from build123d import *

# Parameters (mm, degrees)
SKETCH_1_R      = 0.75
EXTRUDE_1_DEPTH = 15
SKETCH_3_R      = 0.75
EXTRUDE_2_DEPTH = 2
SKETCH_5_R      = 0.75
EXTRUDE_3_DEPTH = 25
SKETCH_7_R      = 0.75
EXTRUDE_4_DEPTH = 5
EXTRUDE_START   = 25
SKETCH_9_R      = 0.75
EXTRUDE_5_DEPTH = 6


with BuildPart() as part:
    # 草图1 → 凸台-拉伸1 (new body)
    with BuildSketch(Plane(origin=(0, 0, 0), x_dir=(1, 0, 0), z_dir=(0, 1, 0))):
        with Locations(Location((0, 0, 0), (0, 0, 270))):
            Circle(SKETCH_1_R)
    extrude(amount=EXTRUDE_1_DEPTH)

    # 草图2 → 旋转1 (revolve)
    with BuildSketch(Plane.XY):
        with BuildLine():
            Line((0, 15.75), (0, 14.25))
            ThreePointArc((0, 14.25), (0.75, 15), (0, 15.75))
        make_face()
    revolve(axis=Axis((0, 15.75, 0), (0, -1, 0)))

    # 草图3 → 凸台-拉伸2 (add)
    with BuildSketch(Plane(origin=(0, 0, 0), x_dir=(0, 0, -1), z_dir=(1, 0, 0))):
        with Locations((0, 15)):
            Circle(SKETCH_3_R)
    extrude(amount=EXTRUDE_2_DEPTH)

    # 草图4 → 旋转2 (revolve)
    with BuildSketch(Plane(origin=(2, 0, 0), x_dir=(0, 0, -1), z_dir=(1, 0, 0))):
        with BuildLine():
            Line((0, 15.75), (0, 14.25))
            ThreePointArc((0, 14.25), (0.75, 15), (0, 15.75))
        make_face()
    revolve(axis=Axis((2, 15.75, 0), (0, -1, 0)))

    # 草图5 → 凸台-拉伸3 (add)
    with BuildSketch(Plane(origin=(0, 15, 0), x_dir=(1, 0, 0), z_dir=(0, 1, 0))):
        with Locations(Location((2, 0, 0), (0, 0, 270))):
            Circle(SKETCH_5_R)
    extrude(amount=EXTRUDE_3_DEPTH)

    # 草图6 → 旋转3 (revolve)
    with BuildSketch(Plane(origin=(0, 40, 0), x_dir=(1, 0, 0), z_dir=(0, 1, 0))):
        with BuildLine():
            Line((2, 0.75), (2, -0.75))
            ThreePointArc((2, -0.75), (2.75, 0), (2, 0.75))
        make_face()
    revolve(axis=Axis((2, 40, -0.75), (0, 0, 1)))

    # 草图7 → 凸台-拉伸4 (add)
    with BuildSketch(Plane(origin=(2, 0, 0), x_dir=(0, 0, -1), z_dir=(1, 0, 0))):
        with Locations((0, 40)):
            Circle(SKETCH_7_R)
    extrude(amount=-EXTRUDE_4_DEPTH)

    # 草图8 → 旋转5 (revolve)
    with BuildSketch(Plane.ZY.offset(3)):
        with BuildLine():
            Line((-0.75, 40), (0.75, 40))
            ThreePointArc((0.75, 40), (0, 40.75), (-0.75, 40))
        make_face()
    revolve(axis=Axis((-3, 40, -0.75), (0, 0, 1)))

    # 草图9 → 凸台-拉伸5 (add)
    with BuildSketch(Plane(origin=(0, 15, 0), x_dir=(1, 0, 0), z_dir=(0, 1, 0)).offset(EXTRUDE_START)):
        with Locations(Location((-3, 0, 0), (0, 0, 270))):
            Circle(SKETCH_9_R)
    extrude(amount=EXTRUDE_5_DEPTH)


solid = part.part
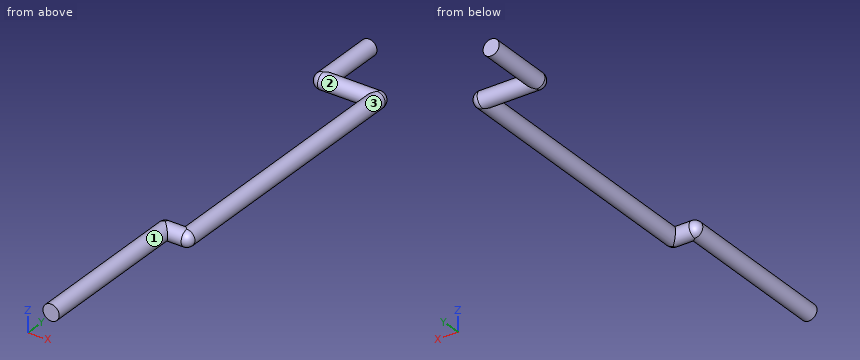
Could you check a few things on this model? Use its own coordinates, in mm. Face numbers are marked on the shaded views. Round coordinates to 2 decimals unless told otherwise and drop trailing zeros. Loops run counter-clockwise (first coordinate to the right, second up) from the corner with the lowest first, then second, coordinate; pieces in that order, holes last. Notation, with made-up numbers: (-28, 77) -> (12, 77) arc R27 ccw to (12, 109) -> close; hole circle Ø1 at (10, -24). An arc over 180 degrees is marked (long way). Use CSV: the item, a comma, the result in double quotes.
(1) Suppose I cut it at C-C on y = 6. Write out the boundary of the cut face in (x, z), plus the area to 3 significant figures.
Return value:
outline,"circle Ø1.5 at (0, 0)"
area,"1.77 mm²"
(2) If we mould it in two halves opening along Y, with no side actions, what happens to the marked faces 1, 2 and 3? For each: +Y half, -Y half, draft (parallel to the pull), parting line (faces both ways), or undercut.
Return value:
face 1,"draft"
face 2,"undercut"
face 3,"undercut"
(3) Suppose I cut it at B-B on x = -1.75. Write out the boundary of the cut face in (y, z).
Return value:
outline,"circle Ø1.5 at (40, 0)"
(4) If I drill on probe 1 along X at (y, z) = (10.5, -0.1); probe 2 along Y at (x, z) = (0.25, -0.6); probe 3 along Y at (x, z) = (0.75, 0.3), over which ranges is the centre line in solid material (lowest first)? Write a range as [from, to].
Return value:
probe 1,"x = [-0.74, 0.74]"
probe 2,"y = [0, 15.45], [39.55, 40.45]"
probe 3,"y = [14.31, 15.69], [39.31, 40.69]"
(5) Suppose I cut it at A-A on z = 0. Write out the boundary of the cut face in (x, y).
Return value:
outline,"(-3.75, 40) arc R0.75 ccw to (-3, 39.25) -> (1.25, 39.25) -> (1.25, 15.75) -> (0, 15.75) arc R0.75 ccw to (-0.75, 15) -> (-0.75, 0) -> (0.75, 0) -> (0.75, 14.25) -> (2, 14.25) arc R0.75 ccw to (2.75, 15) -> (2.75, 40) arc R0.75 ccw to (2, 40.75) -> (-2.25, 40.75) -> (-2.25, 46) -> (-3.75, 46) -> close"
